Read the model definition and answer for the solid it produces. Units are mm, in the model's axes. A direction names the side the tool comes from. Give positions to 0.01 mm unless a question says otherwise; leave off trailing zeros. Order: outer loops, then holes, each group sorted by start corner. A loop starts at its lowest first (then second) coordinate and runs counter-clockwise, first axis right, second up.
Item 1: A cutting plane is placed at D-D (x = 15). Write down the section's boundary in (y, z), plus the area to 3 significant figures.
Item 2: The mould has two halves that part along Y. Classify faces 1 (the face through (-1.08, -42.26, -4.88)), 2 (the face through (-19, -22.845, -9)), 3 (the face through (-0.3, -25, -5.2)): +Y half, -Y half, draft (parallel to the pull), parting line (faces both ways), or undercut.
Item 3: Which of the six approach directions +Z, -Z, +X, -X, +Y, -Y give full straight-line access (tool end or side, diameter ignored) to faces 4 (the face through (-0.1, -60, -2.2)), 5 (the face through (-6.227, -12.362, 19.774))?
Item 4: Find the intervals of material crossed by line 1 along Y through (x, z) = (21, -10.5); line 2 along Z through (x, y) = (0, -19); line 3 along Z through (x, y) = (0, -28), in increasing order.
Item 5: A cutting plane is placed at C-C (y = -50.5). Write down the section's boundary in (x, z), plus the area to 3 significant figures.
Item 6: A cutting plane is placed at A-A (z = 0). Write down the section's boundary in (x, y), plus the area to 3 significant figures.
Item 7: Given pin 1 Ø1.5 at (x, z) = (-2.5, -18.5) entering from -Y; pin 2 Ø8 at (y, z) = (-33.5, -1.5) entering from -X; pin 3 Ø10 at (x, y) = (-4.5, -8.5) entering from -Z, each flat-ended and moving along its own axis, determine where each tip first touches the part or whether it passes through.
Item 8: A cutting plane is placed at B-B (x = 0). Write down the section's boundary in (y, z), plus the area to 3 significant figures.
from build123d import *

# Parameters (mm, degrees)
F0_R     = 25
F0_R_2   = 5
F1_DEPTH = 25
F0_R_3   = 2
F2_DEPTH = 60


with BuildPart() as f1:
    # F0 (on Front) → F1 (new body)
    with BuildSketch(Plane.XZ):
        Circle(F0_R)
        Circle(F0_R_2, mode=Mode.SUBTRACT)
    extrude(amount=F1_DEPTH)

    # F0 (on Front) → F2 (join)
    with BuildSketch(Plane.XZ):
        Circle(F0_R_2)
        Circle(F0_R_3, mode=Mode.SUBTRACT)
    extrude(amount=F2_DEPTH)

    # F3 (on Right) → F4 (revolve, cut)
    with BuildSketch(Plane.YZ):
        Polygon((-2.168103, 20.730987), (-2.168103, 26.635021), (-22.844952, 26.710875), (-22.844952, 20.730987), align=None)
    revolve(axis=Axis((0, -34.338176, 0), (0, -1, 0)), mode=Mode.SUBTRACT)


solid = f1.part
Response values:
1. outline: (-25, -20) - (-22.84, -20) - (-22.84, -14.31) - (-2.17, -14.31) - (-2.17, -20) - (0, -20) - (0, 20) - (-2.17, 20) - (-2.17, 14.31) - (-22.84, 14.31) - (-22.84, 20) - (-25, 20) - close
1. area: 765 mm2
2. face 1: draft
2. face 2: undercut
2. face 3: -Y half
3. face 4: +Z, -Z, +X, -X, -Y
3. face 5: none
4. line 1: y = -25 to -22.84, -2.17 to 0
4. line 2: z = -20.73 to -2, 2 to 20.73
4. line 3: z = -5 to -2, 2 to 5
5. outline: circle Ø10 at (0, 0); hole circle Ø4 at (0, 0)
5. area: 66.0 mm2
6. outline: (-25, -25) - (-5, -25) - (-5, -60) - (-2, -60) - (-2, 0) - (-25, 0) - (-25, -2.17) - (-20.73, -2.17) - (-20.73, -22.84) - (-25, -22.84) - close; (2, -60) - (5, -60) - (5, -25) - (25, -25) - (25, -22.84) - (20.73, -22.84) - (20.73, -2.17) - (25, -2.17) - (25, 0) - (2, 0) - close
6. area: 1,180 mm2
7. pin 1: stops at y = -25
7. pin 2: stops at x = -5
7. pin 3: stops at z = -20.73
8. outline: (-60, -5) - (-25, -5) - (-25, -25) - (-22.84, -25) - (-22.84, -20.73) - (-2.17, -20.73) - (-2.17, -25) - (0, -25) - (0, -2) - (-60, -2) - close; (-60, 2) - (0, 2) - (0, 25) - (-2.17, 25) - (-2.17, 20.73) - (-22.84, 20.73) - (-22.84, 25) - (-25, 25) - (-25, 5) - (-60, 5) - close
8. area: 1,180 mm2
